```python
from build123d import *

# Parameters (mm, degrees)
EXTRUSION1_DEPTH        = 3
ESQUISSE2_W             = 50
ESQUISSE2_H             = 6
ENL_V_MAT_EXTRU_1_DEPTH = 6
CONG_1_R                = 5


with BuildPart() as part:
    # Esquisse1 → Extrusion1 (new body)
    with BuildSketch(Plane.XY):
        Polygon((-63.845510563, 55.495422535), (-53.845510563, 55.495422535), (-53.845510563, 11.495422535), (6.154489437, 11.495422535), (6.154489437, 55.495422535), (16.154489437, 55.495422535), (16.154489437, -4.504577465), (-63.845510563, -4.504577465), align=None)
    extrude(amount=EXTRUSION1_DEPTH)

    # Esquisse2 → Enlèv. mat.-Extru.1 (cut)
    with BuildSketch(Plane.XY.offset(3)):
        with Locations((-23.845510563, 3.495422535)):
            Rectangle(ESQUISSE2_W, ESQUISSE2_H)
    extrude(amount=-ENL_V_MAT_EXTRU_1_DEPTH, mode=Mode.SUBTRACT)

    # Congé1
    cong_1_edges = [part.edges().sort_by_distance(p)[0] for p in [
        (-53.845510563, 11.495422535, 1.5),
        (6.154489437, 11.495422535, 1.5),
        (16.154489437, 55.495422535, 1.5),
        (6.154489437, 55.495422535, 1.5),
        (-53.845510563, 55.495422535, 1.5),
        (-63.845510563, 55.495422535, 1.5),
        (16.154489437, -4.504577465, 1.5),
        (-63.845510563, -4.504577465, 1.5),
    ]]
    fillet(cong_1_edges, radius=CONG_1_R - 0.0001)  # a hair under: the kernel refuses the full size


solid = part.part
```
The listing builds one solid part. Answer for the finished solid, in the listing's coordinates (mm). A direction names the side the tool comes from. Round coordinates to 2 decimals unless told otherwise and drop trailing zeros. Loops run counter-clockwise (first coordinate to the right, second up) from the corner with the lowest first, then second, coordinate; pieces in that order, holes last.
1) A cutting plane is placed at C-C on y = 38.5. Determine the outline of the cut face in (x, z), plus the area to 3 significant figures.
Outcome:
outline: (-63.85, 0) - (-53.85, 0) - (-53.85, 3) - (-63.85, 3) - close; (6.15, 0) - (16.15, 0) - (16.15, 3) - (6.15, 3) - close
area: 60.0 mm2
2) For faces 1 (the face through (-53.846, 34, 1)), 2 (the face through (-21, 10, 0)), 3 (the face through (1.154, 3, 2)), determine the directions among +Z, -Z, +X, -X, +Y, -Y from which every point of the face is accessible in a straight line to the end or side of a thin tool.
Outcome:
face 1: +Z, -Z, +Y
face 2: -Z, +X, -X, +Y, -Y
face 3: +Z, -Z
3) A cutting plane is placed at D-D on x = -55.5. Determine the outline of the cut face in (y, z), plus the area to 3 significant figures.
Outcome:
outline: (-4.5, 0) - (54.21, 0) - (54.21, 3) - (-4.5, 3) - close
area: 176 mm2
4) A cutting plane is placed at B-B on x = -11.5. Determine the outline of the cut face in (y, z).
Outcome:
outline: (-4.5, 0) - (0.5, 0) - (0.5, 3) - (-4.5, 3) - close; (6.5, 0) - (11.5, 0) - (11.5, 3) - (6.5, 3) - close
5) For a pull along Y with two mould halves and no side action, classify faces 4 (the face through (-21, 10, 3)), 5 (the face through (-48.846, 3, 2)), 6 (the face through (4.65, 12.92, 1.52)), 7 (the face through (-24, 0.495, 2)) as released by +Y, released by -Y, zero draft, split by the parting line, or undercut.
Outcome:
face 4: zero draft
face 5: undercut
face 6: released by +Y
face 7: undercut
6) Given P1, Ø1.5, axis at x = -22.5, z = 2, coming from the +Y side; P2, Ø12, axis at x = -17, y = 12, coming from the +Z side, each flat-ended and moving along its own axis, determine where each tip first touches the part or whether it passes through.
Outcome:
P1: stops at y = 11.5
P2: stops at z = 3
7) Consider line 1 (X direction, y = 50.5, z = 1.8); line 2 (Y direction, x = -10.5, z = 2.7); line 3 (X direction, y = 4.5, z = 1.45). Determine where each line is inside the solid, lowest interval first.
Outcome:
line 1: x = -63.85 to -53.85, 6.15 to 16.15
line 2: y = -4.5 to 0.5, 6.5 to 11.5
line 3: x = -63.85 to -48.85, 1.15 to 16.15
